The listing builds one solid part. Answer for the finished solid, in the listing's coordinates (mm). Face numbers are marked on the shaded views. A direction names the side the tool comes from. Round coordinates to 2 decimals unless told otherwise and drop trailing zeros. Loops run counter-clockwise (first coordinate to the right, second up) from the corner with the lowest first, then second, coordinate; pieces in that order, holes last. Notation, with made-up numbers: (44.5, 4) - (94.5, 4) arc R24 ccw to (94.5, 23) - close; hole circle Ø11 at (88.25, 20). An arc over 180 degrees is marked (long way). Write item = value, one per line. Start each with the question number.
1) Section B-B, the plane z = 27 is taken. Determine the outline of the cut face in (x, y).
2) Straight lines are drawn through the part: line 1 along X through (y, z) = (-15, 27); line 2 along X through (y, z) = (3, -3); line 3 along Z through (x, y) = (11.5, 0.5). For each, find the intervals that lie inside material, in ascending order.
3) Section A-A, the plane y = 3.75 is taken. Determine the outline of the cut face in (x, z), and give its area (3 significant figures).
4) Section C-C, the plane x = -22.5 is taken. Determine the outline of the cut face in (y, z), and give its area (3 significant figures).
5) For a pull along X with two mould halves and no side action, classify the marked faces 3, 4, 5 and 6 as released by +X, released by -X, zero draft, split by the parting line, or undercut.
6) Section D-D, the plane y = 12.5 is taken. Determine the outline of the cut face in (x, z).
7) A tool of negligible diameter and unlimited length cuts with its end or side. For the marked faces 1 and 2, from which of +Z, -Z, +X, -X, +Y, -Y can it reach the whole face along a straight path? Write none if from no direction.
8) Given pin 1 Ø13 at (x, y) = (22.5, 3.75) entering from +Z; pin 2 Ø5 at (x, z) = (23, 5.5) entering from +Y; pin 3 Ø13 at (x, z) = (22.5, 27) entering from +Y, each flat-ended and moving along its own axis, determine where each tip first touches the part or whether it passes through.
from build123d import *

# Parameters (mm, degrees)
SZKIC1_R                    = 4
DODANIE_WYCI_GNI_CIE1_DEPTH = 5
SZKIC2_W                    = 65
SZKIC2_H                    = 47
SZKIC2_R                    = 4
DODANIE_WYCI_GNI_CIE2_DEPTH = 5
ZAOKR_GLENIE1_R             = 5
ZAOKR_GLENIE2_R             = 5


with BuildPart() as part:
    # Szkic1 → Dodanie-wyciągnięcie1 (new body)
    with BuildSketch(Plane.XY):
        with BuildLine():
            Line((17.860571099, 18), (32.5, 18))
            Line((32.5, 18), (32.5, -18))
            Line((32.5, -18), (-32.5, -18))
            Line((-32.5, -18), (-32.5, 18))
            Line((-32.5, 18), (-17.860571099, 18))
            ThreePointArc((-17.860571099, 18), (0, 7), (17.860571099, 18))
        make_face()
        with Locations((-22.5, 3.75)):
            Circle(SZKIC1_R, mode=Mode.SUBTRACT)
        with Locations(Location((22.5, 3.75, 0), (0, 0, 180))):
            Circle(SZKIC1_R, mode=Mode.SUBTRACT)
    extrude(amount=-DODANIE_WYCI_GNI_CIE1_DEPTH)

    # Szkic2 → Dodanie-wyciągnięcie2 (add)
    with BuildSketch(Plane.XZ.offset(18)):
        with Locations((0, 18.5)):
            Rectangle(SZKIC2_W, SZKIC2_H)
        with Locations(Location((-22.5, 27, 0), (0, 0, 270))):
            Circle(SZKIC2_R, mode=Mode.SUBTRACT)
        with Locations(Location((22.5, 27, 0), (0, 0, 90))):
            Circle(SZKIC2_R, mode=Mode.SUBTRACT)
    extrude(amount=-DODANIE_WYCI_GNI_CIE2_DEPTH)

    # Zaokrąglenie1
    zaokr_glenie1_edges = [part.edges().sort_by_distance(p)[0] for p in [
        (0, -13, 0),
    ]]
    fillet(zaokr_glenie1_edges, radius=ZAOKR_GLENIE1_R)

    # Zaokrąglenie2
    zaokr_glenie2_edges = [part.edges().sort_by_distance(p)[0] for p in [
        (0, -18, -5),
    ]]
    fillet(zaokr_glenie2_edges, radius=ZAOKR_GLENIE2_R)


solid = part.part
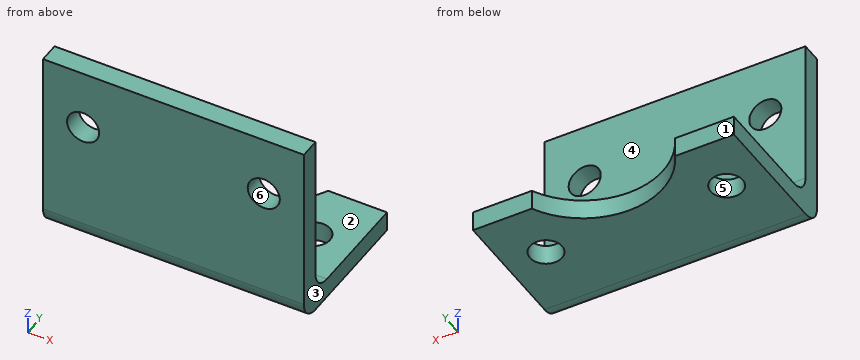
Geometry check:
q1.outline = (-32.5, -18) - (-26.5, -18) - (-26.5, -13) - (-32.5, -13) - close; (-18.5, -18) - (18.5, -18) - (18.5, -13) - (-18.5, -13) - close; (26.5, -18) - (32.5, -18) - (32.5, -13) - (26.5, -13) - close
q2.line_1 = -32.5 to -26.5, -18.5 to 18.5, 26.5 to 32.5
q2.line_2 = -32.5 to -26.43, -18.57 to 18.57, 26.43 to 32.5
q2.line_3 = -5 to 0
q3.outline = (-32.5, -5) - (-26.5, -5) - (-26.5, 0) - (-32.5, 0) - close; (-18.5, -5) - (18.5, -5) - (18.5, 0) - (-18.5, 0) - close; (26.5, -5) - (32.5, -5) - (32.5, 0) - (26.5, 0) - close
q3.area = 245 mm2
q4.outline = (-18, 0) arc R5 ccw to (-13, -5) - (-0.25, -5) - (-0.25, 0) - (-8, 0) arc R5 cw to (-13, 5) - (-13, 23) - (-18, 23) - close; (-18, 31) - (-13, 31) - (-13, 42) - (-18, 42) - close; (7.75, -5) - (18, -5) - (18, 0) - (7.75, 0) - close
q4.area = 310 mm2
q5.face_3 = released by +X
q5.face_4 = zero draft
q5.face_5 = undercut
q5.face_6 = undercut
q6.outline = (-32.5, -5) - (-13.77, -5) - (-13.77, 0) - (-32.5, 0) - close; (13.77, -5) - (32.5, -5) - (32.5, 0) - (13.77, 0) - close
q7.face_1 = +Z, -Z, +X, -X, +Y
q7.face_2 = +Z, +X, -X, +Y
q8.pin_1 = 0
q8.pin_2 = -12.58
q8.pin_3 = -13
